Autodesk Inventor part; units mm, degrees
ref_plane "Work Plane1" through (29, 0, 0) normal (0, -1, 0) x (1, 0, 0)
ref_plane "YZ Plane" through (0, 0, 0) normal (1, 0, 0) x (0, 1, 0)
ref_plane "XZ Plane" through (0, 0, 0) normal (0, 1, 0) x (-1, 0, 0)
sketch "Sketch1" plane through (0, 0, 0) normal (0, 0, 1) x (1, 0, 0)
  line L0 (-0.0931, 0) -> (9.525, 0)
  line L1 (9.525, 0) -> (9.525, 2.0828)
  line L2 (9.525, 2.0828) -> (1.5902, 2.0828)
  line L3 (1.5902, 2.0828) -> (0.0001, 2.0828)
  line L4 (0.0001, 2.0828) -> (0, 2.0828)
  line L5 (0, 2.0828) -> (0, 3.9624)
  line L6 (0, 3.9624) -> (-2.2098, 3.9624)
  line L7 (-2.2098, 3.9624) -> (-2.2098, 1.3785)
  line L8 (-2.2098, 1.3785) -> (-0.889, 1.3785)
  line L9 (-0.889, 1.3785) -> (-0.0931, 0)
  line L10 (-4.5568, 0) -> (11.872, 0)
  line L11 (0, -0.7925) -> (0, 4.7549)
  line L12 (1.5902, 2.0828) -> (0, 2.0828) construction
  dimension "d1" = 7.9348
  dimension "d2" = 1.5901
  dimension "d3" = 2.2098
  dimension "d4" = 1.3208
  dimension "d5" = 60
  dimension "d6" = 4.1656
  dimension "d7" = 4.1656
  dimension "d8" = 2.757
  dimension "d9" = 7.9248
  dimension "d26" = 9.525
revolve "Body" add sketch "Sketch1" angle 360 about axis through (-0.0931, 0, 0) along (1, 0, 0)
sketch "Sketch2" plane through (-2.2098, 0, 0) normal (-1, 0, 0) x (0, 0, 1)
  circle A0 centre (0, 0) radius 1.3785
  line L0 (0, -5.5474) -> (0, 5.5474)
  line L1 (-5.5474, 0) -> (5.5474, 0)
  line L2 (1.3785, 0) -> (0.6892, -1.1938)
  line L3 (0.6892, -1.1938) -> (-0.6892, -1.1938)
  line L4 (-0.6892, -1.1938) -> (-1.3785, 0)
  line L5 (-1.3785, 0) -> (-0.6892, 1.1938)
  line L6 (-0.6892, 1.1938) -> (0.6892, 1.1938)
  line L7 (0.6892, 1.1938) -> (1.3785, 0)
extrude "Slot" add sketch "Sketch2" against normal up to next contours L7 A0 | A0 L2 | L6 L0 A0 | A0 L0 L3 | L0 L6 A0 | A0 L3 L0 | L4 A0 | A0 L5
fillet "Fillet1" radius 1.9558 1 edges at (-2.2098, -3.9624, 0)
thread "Thread"
chamfer "Chamfer1" distance 0.4869 distance2 0.4869 1 edges at (9.525, -2.0828, 0) measured on face at (9.525, -0.1898, 0.4203)
ref_plane "Work Plane1" through (29, 0, 0) normal (0, -1, 0) x (1, 0, 0)
fillet "Fillet2" radius 0.1 1 edges at (0.0001, -2.0828, 0)
equation "\"d30\" = R"
equation "\"d17\" = RR"
equation "\"d13\" = GEL"
equation "\"d15\" = -0.5 * SPD + 0.5 * GD"
equation "\"d16\" = GUL"
equation "\"d1\" = GEL"
equation "\"d3\" = KOH"
equation "\"d4\" = INTI"
equation "\"d6\" = GD"
equation "\"d7\" = BDM"
equation "\"d8\" = 1.1547 * SW"
equation "\"d9\" = KOD"
equation "\"d26\" = NLG"
equation "\"GD\" = NND"
equation "\"NLG\" = 9.525"
equation "\"GEL\" = 7.93476"
equation "\"KOD\" = 7.9248"
equation "\"KOH\" = 2.2098"
equation "\"INTI\" = 1.3208"
equation "\"GAL\" = 1.59004"
equation "\"GUL\" = 0.48692"
equation "\"BDM\" = NND"
equation "\"SW\" = 2.3876"
equation "\"RR\" = 1.9558"
equation "\"SPD\" = 3.19176"
equation "\"R\" = 0.1"
equation "\"TOA\" = 30deg"
equation "\"GD1\" = SPD"
equation "\"THREADDIA\" = 4.1656"
equation "\"KOH1\" = 0.381"
equation "\"NND\" = 4.1656"
equation "\"E0\" = 2.75768"
properties part number "ANSI B18.3 - 8 - 32 x 3/8" material "Steel, Mild"
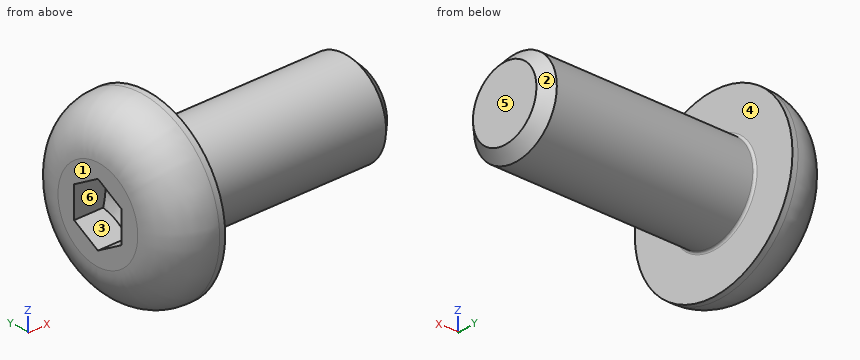
Could you check a few things on this model? Use its own coordinates, in mm. Face numbers are marked on the shaded views. A direction names the side the tool comes from. Coordinates: 2 decimals unless noted, no trailing zeros. Order: outer loops, then holes, each group sorted by start corner. A loop starts at its lowest first (then second) coordinate and runs counter-clockwise, first axis right, second up. Notation, with made-up numbers: M 65,-1 L 115,-1 A16 ccw 115,27 Z; hole C 65.5,56 d10. An arc over 180 degrees is marked long. Use a Markdown table: item, result. Add a question column.
Q1. I'm going to push flat-ended pins straight in: pin 1 (1 mm diameter, centred on y = -2.5, z = -1.5, fed in from -X); pin 2 (0.7 mm diameter, centred on x = -1.5, z = 0, fed in from -Y); pin 3 (1.5 mm diameter, centred on x = -1.5, z = 0, fed in from +Y). Where does each tip first touch, or does it pass through?
Q2. I want a section at A-A on x = 1.25. List the corners of the cut face in (y, z) for me, then the cut area to 3 significant figures.
Q3. If I drill on L1, parallel to Z at x = 2.75, y = 0; L2, parallel to Y at x = -1.5, z = 0.5, over which ranges is the centre line in solid material (lowest first)?
Q4. We'd pull the mould along Y, two halves only. Please class the marked faces 1, 2 and 3: pulls with the +Y half, pulls with the -Y half, needs draft (parallel to the pull), parting line crosses it, or undercut.
Q5. Which directions (+Z, -Z, +X, -X, +Y, -Y) give clear straight access to the entire face, cutting with the end or side of a thin tool? Please do the marked faces 4, 5 and 6.
Checked values:
| question | item | result |
|---|---|---|
| 1 | pin 1 | x = -2.17 |
| 1 | pin 2 | y = -3.75 |
| 1 | pin 3 | y = 3.9 |
| 2 | outline | C 0,0 d4.17 |
| 2 | area | 13.6 mm² |
| 3 | L1 | -2.08 to 2.08 |
| 3 | L2 | -3.48 to -1.19, 1.19 to 3.48 |
| 4 | face 1 | needs draft |
| 4 | face 2 | parting line crosses it |
| 4 | face 3 | undercut |
| 5 | face 4 | +X |
| 5 | face 5 | +Z, -Z, +X, +Y, -Y |
| 5 | face 6 | -X |
